Read the model definition and answer for the solid it produces. Units are mm, in the model's axes. A direction names the side the tool comes from. Give positions to 0.01 mm unless a question says otherwise; leave off trailing zeros. Loops run counter-clockwise (first coordinate to the right, second up) from the corner with the lowest first, then second, coordinate; pieces in that order, holes last. Notation, with made-up numbers: (21, 69) -> (51, 69) arc R18 cw to (51, 94) -> close; hole circle Ø2 at (56.25, 55.25). An arc over 180 degrees is marked (long way). Write each question's results on one line, items separated by ' | '. Start each with the question number.
Item 1: Section B-B on z = 22 is taken. Write down the section's boundary in (x, y).
Item 2: Section A-A on y = 6.15 is taken. Write down the section's boundary in (x, z) (3 decimals).
Item 3: Which of the six approach directions +Z, -Z, +X, -X, +Y, -Y give full straight-line access (tool end or side, diameter ignored) to faces 1 (the cylindrical face through (3.375, 42.821, 38.286)), 2 (the flat face through (13, 0, 22)), 3 (the cylindrical face through (1.479, 7.499, 6.735))?
Item 4: Section D-D on y = 38.15 is taken. Write down the section's boundary in (x, z) (3 decimals), and give its area (3 significant figures).
Item 5: Determine the mould class of faces 4 (the cylindrical face through (1.48, 36.73, 38.61)), 5 (the flat face through (10, 18, 0)), 6 (the flat face through (4, 41.3, 37)), 7 (the cylindrical face through (1.479, 7.736, 37.667)) for opening direction Y: +Y half, -Y half, draft (parallel to the pull), parting line (faces both ways), or undercut.
Item 6: Each of these flat-tipped pins is pushed along its axis until it touches: P1, Ø5, axis at y = 6.15, z = 37.875, coming from the +X side; P2, Ø2, axis at y = 4.5, z = 28, coming from the +X side; P3, Ø2.5, axis at y = 38.15, z = 5.875, coming from the +X side (3 decimals). Where does it stop, or does it pass through?
Item 7: Find the intervals of material crossed by line 1 (X direction, y = 12.5, z = 26.5); line 2 (X direction, y = 18, z = 7.5); line 3 (Y direction, x = 9, z = 34), in increasing order.
Item 8: Section C-C on x = 24.25 is taken. Write down the section's boundary in (y, z), and give its area (3 significant figures).
```python
from build123d import *

# Parameters (mm, degrees)
BOSS_EXTRUDE1_DEPTH = 43.75
SKETCH2_R           = 1.6
CUT_EXTRUDE1_DEPTH  = 3
SKETCH3_R           = 1.5
CUT_EXTRUDE2_DEPTH  = 3


with BuildPart() as part:
    # Sketch1 → Boss-Extrude1 (new body)
    with BuildSketch(Plane.XY):
        Polygon((0, 0), (0, 44.3), (8.25, 44.3), (26, 0), align=None)
    extrude(amount=BOSS_EXTRUDE1_DEPTH)

    # Sketch2 → Cut-Extrude1 (cut)
    with BuildSketch(Plane.ZY):
        with Locations((5.875, 38.15)):
            Circle(SKETCH2_R)
        with Locations((37.875, 38.15)):
            Circle(SKETCH2_R)
        with Locations((5.875, 6.15)):
            Circle(SKETCH2_R)
        with Locations((37.875, 6.15)):
            Circle(SKETCH2_R)
    extrude(amount=-CUT_EXTRUDE1_DEPTH, mode=Mode.SUBTRACT)

    # Sketch3 → Cut-Extrude2 (cut)
    with BuildSketch(Plane(origin=(0, 44.3, 0), x_dir=(1, 0, 0), z_dir=(0, 1, 0))):
        with Locations(Location((3.95, -7.3, 0), (0, 0, 270))):
            Circle(SKETCH3_R)
        with Locations(Location((3.95, -36.9, 0), (0, 0, 270))):
            Circle(SKETCH3_R)
    extrude(amount=-CUT_EXTRUDE2_DEPTH, mode=Mode.SUBTRACT)


solid = part.part
```
Findings:
1) outline: (0, 0) -> (26, 0) -> (8.25, 44.3) -> (0, 44.3) -> close
2) outline: (0, 0) -> (23.536, 0) -> (23.536, 43.75) -> (0, 43.75) -> (0, 39.475) -> (3, 39.475) -> (3, 36.275) -> (0, 36.275) -> (0, 7.475) -> (3, 7.475) -> (3, 4.275) -> (0, 4.275) -> close
3) face 1: +Y | face 2: +Z, -Z, +X, -X, -Y | face 3: -X
4) outline: (0, 0) -> (10.714, 0) -> (10.714, 43.75) -> (0, 43.75) -> (0, 39.475) -> (3, 39.475) -> (3, 36.275) -> (0, 36.275) -> (0, 7.475) -> (3, 7.475) -> (3, 4.275) -> (0, 4.275) -> close | area: 450 mm2
5) face 4: undercut | face 5: draft | face 6: +Y half | face 7: undercut
6) P1: x = 24.54 | P2: x = 24.6 | P3: x = 11.215
7) line 1: 0 to 20.99 | line 2: 0 to 18.79 | line 3: 0 to 42.43
8) outline: (0, 0) -> (4.37, 0) -> (4.37, 43.75) -> (0, 43.75) -> close | area: 191 mm2
